Autodesk Inventor part; units mm, degrees
ref_plane "YZ Plane" through (0, 0, 0) normal (1, 0, 0) x (0, 1, 0)
ref_plane "XZ Plane" through (0, 0, 0) normal (0, 1, 0) x (-1, 0, 0)
ref_plane "XY Plane" through (0, 0, 0) normal (0, 0, 1) x (1, 0, 0)
sketch "Sketch1" plane through (0, 0, 0) normal (0, 0, 1) x (1, 0, 0)
  line L0 (0, 0) -> (50.8, 0)
  line L1 (50.8, 0) -> (50.8, 50.8)
  line L2 (50.8, 50.8) -> (0, 50.8)
  line L3 (0, 50.8) -> (0, 0)
  dimension "d0" = 50.8
  dimension "d1" = 50.8
extrude "Extrusion1" add sketch "Sketch1" along normal blind 50.8
sketch "Sketch2" plane through (0, 50.8, 0) normal (0, 1, 0) x (1, 0, 0)
  line L0 (50.8, 0) -> (0, 0)
  line L1 (0, 0) -> (0, -50.8)
  line L2 (50.8, -50.8) -> (0, -50.8)
  line L3 (50.8, 0) -> (50.8, -50.8)
  line L4 (46.99, -46.99) -> (34.29, -46.99)
  line L5 (34.29, -46.99) -> (34.29, -34.29)
  line L6 (34.29, -34.29) -> (46.99, -34.29)
  line L7 (46.99, -34.29) -> (46.99, -46.99)
  line L8 (19.05, -46.99) -> (19.05, -34.29)
  line L9 (19.05, -34.29) -> (31.75, -34.29)
  line L10 (31.75, -34.29) -> (31.75, -46.99)
  line L11 (31.75, -46.99) -> (19.05, -46.99)
  line L12 (3.81, -46.99) -> (3.81, -34.29)
  line L13 (3.81, -34.29) -> (16.51, -34.29)
  line L14 (16.51, -34.29) -> (16.51, -46.99)
  line L15 (16.51, -46.99) -> (3.81, -46.99)
  line L16 (34.29, -31.75) -> (34.29, -19.05)
  line L17 (34.29, -19.05) -> (46.99, -19.05)
  line L18 (46.99, -19.05) -> (46.99, -31.75)
  line L19 (46.99, -31.75) -> (34.29, -31.75)
  line L20 (19.05, -31.75) -> (19.05, -19.05)
  line L21 (19.05, -19.05) -> (31.75, -19.05)
  line L22 (31.75, -19.05) -> (31.75, -31.75)
  line L23 (31.75, -31.75) -> (19.05, -31.75)
  line L24 (3.81, -31.75) -> (3.81, -19.05)
  line L25 (3.81, -19.05) -> (16.51, -19.05)
  line L26 (16.51, -19.05) -> (16.51, -31.75)
  line L27 (16.51, -31.75) -> (3.81, -31.75)
  line L28 (34.29, -16.51) -> (34.29, -3.81)
  line L29 (34.29, -3.81) -> (46.99, -3.81)
  line L30 (46.99, -3.81) -> (46.99, -16.51)
  line L31 (46.99, -16.51) -> (34.29, -16.51)
  line L32 (19.05, -16.51) -> (19.05, -3.81)
  line L33 (19.05, -3.81) -> (31.75, -3.81)
  line L34 (31.75, -3.81) -> (31.75, -16.51)
  line L35 (31.75, -16.51) -> (19.05, -16.51)
  line L36 (3.81, -16.51) -> (3.81, -3.81)
  line L37 (3.81, -3.81) -> (16.51, -3.81)
  line L38 (16.51, -3.81) -> (16.51, -16.51)
  line L39 (16.51, -16.51) -> (3.81, -16.51)
  dimension "d4" = 12.7
  dimension "d5" = 12.7
  dimension "d6" = 3.81
  dimension "d7" = 3.81
  dimension "d10" = 15.24
  dimension "d13" = 15.24
extrude "Extrusion2" cut sketch "Sketch2" against normal through all contours L4 L5 L6 L7 | L8 L9 L10 L11 | L12 L13 L14 L15 | L16 L17 L18 L19 | L20 L21 L22 L23 | L24 L25 L26 L27 | L28 L29 L30 L31 | L32 L33 L34 L35 | L36 L37 L38 L39
properties part number "Gold" material "UHMW, Black"
Input: part model. Units: mm. Frame: model coordinates. Give positions to 0.01 mm unless a question says otherwise; leave off trailing zeros. Order: outer loops, then holes, each group sorted by start corner. A loop starts at its lowest first (then second) coordinate and runs counter-clockwise, first axis right, second up. Notation, with made-up numbers: M 43,79.5 L 54,79.5 A23 cw 54,93.5 Z; hole C -30.75,42 d5. An arc over 180 degrees is marked long. One line per question, with ' | ' between items.
1) Contact query for flat-ended pins moving along their axis: P1, Ø1.5, axis at y = 42, z = 17, coming from the -X side; P2, Ø1.5, axis at x = 22, z = 14, coming from the +Y side. Output: stop coordinate, or through.
Filled in:
P1: stops at x = 0 | P2: passes through
2) Section B-B on z = 45.5. Output: boundary loops of the cut face in (x, y).
Filled in:
outline: M 0,0 L 3.81,0 L 3.81,50.8 L 0,50.8 Z; M 16.51,0 L 19.05,0 L 19.05,50.8 L 16.51,50.8 Z; M 31.75,0 L 34.29,0 L 34.29,50.8 L 31.75,50.8 Z; M 46.99,0 L 50.8,0 L 50.8,50.8 L 46.99,50.8 Z
3) Draft query along Z for faces 1 (the face through (41, 26, 16.51)), 2 (the face through (41, 26, 46.99)), 3 (the face through (25, 26, 50.8)). Return one class per face: pulls with the +Z half, pulls with the -Z half, needs draft (parallel to the pull), parting line crosses it, or undercut.
Filled in:
face 1: undercut | face 2: undercut | face 3: pulls with the +Z half
4) Section A-A on x = 23.5. Output: boundary loops of the cut face in (y, z).
Filled in:
outline: M 0,0 L 50.8,0 L 50.8,3.81 L 0,3.81 Z; M 0,16.51 L 50.8,16.51 L 50.8,19.05 L 0,19.05 Z; M 0,31.75 L 50.8,31.75 L 50.8,34.29 L 0,34.29 Z; M 0,46.99 L 50.8,46.99 L 50.8,50.8 L 0,50.8 Z
5) Section C-C on y = 23. State how many separate pieces and enclosed holes the cut face has, and give its area (3 significant figures).
Filled in:
separate pieces: 1 | enclosed holes: 9 | area: 1,130 mm2
6) Ray query, L1, parallel to Z at x = 5.5, y = 3.5. Return the intervals inside material, ascending.
Filled in:
L1: z = 0 to 3.81, 16.51 to 19.05, 31.75 to 34.29, 46.99 to 50.8
